```python
from build123d import *

# Parameters (mm, degrees)
BASE_FLANGE1_DEPTH = 355.6
SKETCH6_W          = 25.4
SKETCH6_H          = 152.4
CUT_EXTRUDE1_DEPTH = 533.597507197


# Sheet-metal steps are written as plain solids
with BuildPart() as part:
    # Sketch1 → Base-Flange1 (new body)
    with BuildSketch(Plane(origin=(0, 0, 0), x_dir=(0, 0, -1), z_dir=(1, 0, 0))):
        with BuildLine():
            Line((0, 0), (-290.758180239, 0))
            ThreePointArc((-290.758180239, 0), (-291.920230239, 0.311370359), (-292.77090988, 1.16205))
            Line((-292.77090988, 1.16205), (-409.417574699, 203.2))
            Line((-409.417574699, 203.2), (-408.042759371, 203.99375))
            Line((-408.042759371, 203.99375), (-291.396094552, 1.9558))
            ThreePointArc((-291.396094552, 1.9558), (-291.126480239, 1.686185688), (-290.758180239, 1.5875))
            Line((-290.758180239, 1.5875), (0, 1.5875))
            Line((0, 1.5875), (0, 0))
        make_face()
    extrude(amount=-BASE_FLANGE1_DEPTH)

    # Sketch6 → Cut-Extrude1 (cut, through all)
    with BuildSketch(Plane(origin=(0, -126.483010223, 219.075), x_dir=(1, 0, 0), z_dir=(0, -0.4999999999999979, 0.8660254037844399))):
        with Locations((-177.8, 304.485149399)):
            Rectangle(SKETCH6_W, SKETCH6_H)
    extrude(amount=-CUT_EXTRUDE1_DEPTH, mode=Mode.SUBTRACT)


solid = part.part
```
The model under review builds one solid part; all positions refer to its coordinate system, in mm. A direction names the side the tool comes from. Round coordinates to 2 decimals unless told otherwise and drop trailing zeros. Order: outer loops, then holes, each group sorted by start corner. A loop starts at its lowest first (then second) coordinate and runs counter-clockwise, first axis right, second up.
(1) Take a section at A-A, the plane z = 354.5. State the section outline as (x, y) points, plus the area to 3 significant figures.
Working result:
outline: (-355.6, 108.08) - (-190.5, 108.08) - (-190.5, 111.25) - (-355.6, 111.25) - close; (-165.1, 108.08) - (0, 108.08) - (0, 111.25) - (-165.1, 111.25) - close
area: 1,050 mm2
(2) For P1, Ø1.5, axis at x = -105, y = 152.5, coming from the -Z side; P2, Ø4, axis at x = -60.5, z = 98, coming from the +Y side; P3, Ø12, axis at x = -58.5, y = 39.5, coming from the -Z side, all flat-tipped, find the tip position at first contact; note any pin that passes through.
Working result:
P1: stops at z = 377.88
P2: stops at y = 1.59
P3: stops at z = 309.61
(3) Mouldability with a two-part tool opening along X and no side actions: class faces 1 (the face through (-165.1, 137, 370)), 2 (the face through (-135.8, 100.77, 350.28)), 3 (the face through (-190.5, 137, 370)) as released by +X, released by -X, zero draft, split by the parting line, or undercut.
Working result:
face 1: undercut
face 2: zero draft
face 3: undercut
(4) Take a section at C-C, the plane y = 164. State the section outline as (x, z) points.
Working result:
outline: (-355.6, 384.95) - (-190.5, 384.95) - (-190.5, 386.79) - (-355.6, 386.79) - close; (-165.1, 384.95) - (0, 384.95) - (0, 386.79) - (-165.1, 386.79) - close
(5) Take a section at B-B, the plane x = -170.5. State the section outline as (y, z) points.
Working result:
outline: (0, 0) - (1.59, 0) - (1.59, 290.76) arc R0.74 cw to (1.96, 291.4) - (72.01, 331.84) - (71.22, 333.22) - (1.16, 292.77) arc R2.32 ccw to (0, 290.76) - close
(6) Wall thickness on L1, parallel to Y at x = -18.5, z = 81; L2, parallel to Z at x = -297.5, y = 178.5; L3, parallel to Y at x = -25, z = 381: over which ranges is each line inside the solid? List them lowest first.
Working result:
L1: y = 0 to 1.59
L2: z = 393.32 to 395.16
L3: y = 153.98 to 157.15
(7) Tool access review of faces 4 (the face through (-175, 1.588, 147)), 5 (the face through (-175, 0, 143)): name each direction out of +Z, -Z, +X, -X, +Y, -Y from which nothing blocks a thin tool from reaching the whole face with its end or side.
Working result:
face 4: -Z, +X, -X, +Y
face 5: +Z, -Z, +X, -X, -Y
(8) Take a section at D-D, the plane z = 285.5. State the section outline as (x, y) points, plus the area to 3 significant figures.
Working result:
outline: (-355.6, 0) - (0, 0) - (0, 1.59) - (-355.6, 1.59) - close
area: 565 mm2
